```python
from build123d import *

# Parameters (mm, degrees)
SKETCH2_R           = 3
BOSS_EXTRUDE1_DEPTH = 5
SKETCH3_R           = 1.5
BOSS_EXTRUDE2_DEPTH = 5
CUT_EXTRUDE1_START  = -2.5
CUT_EXTRUDE1_DEPTH  = 2.5


with BuildPart() as part:
    # Sketch2 → Boss-Extrude1 (new body)
    with BuildSketch(Plane(origin=(0, 0, 0), x_dir=(1, 0, 0), z_dir=(0, 1, 0))):
        with Locations(Location((0, 0, 0), (0, 0, 270))):
            Circle(SKETCH2_R)
    extrude(amount=BOSS_EXTRUDE1_DEPTH)

    # Sketch3 → Boss-Extrude2 (add)
    with BuildSketch(Plane(origin=(0, 5, 0), x_dir=(1, 0, 0), z_dir=(0, 1, 0))):
        with Locations(Location((0, 0, 0), (0, 0, 270))):
            Circle(SKETCH3_R)
    extrude(amount=BOSS_EXTRUDE2_DEPTH)

    # Sketch4 → Cut-Extrude1 (cut)
    with BuildSketch(Plane(origin=(0, 10, 0), x_dir=(1, 0, 0), z_dir=(0, 1, 0)).offset(CUT_EXTRUDE1_START)):
        with BuildLine():
            Line((-1.456893676, -0.357016549), (1.456893676, -0.357016549))
            ThreePointArc((1.456893676, -0.357016549), (0, -1.5), (-1.456893676, -0.357016549))
        make_face()
    extrude(amount=CUT_EXTRUDE1_DEPTH, mode=Mode.SUBTRACT)


solid = part.part
```
Input: part model. Units: mm. Frame: model coordinates. A direction names the side the tool comes from. Round coordinates to 2 decimals unless told otherwise and drop trailing zeros. Loops run counter-clockwise (first coordinate to the right, second up) from the corner with the lowest first, then second, coordinate; pieces in that order, holes last. Notation, with made-up numbers: (11.5, 57) - (51.5, 57) arc R13 cw to (51.5, 75) - close; hole circle Ø2 at (-26, -6.75). An arc over 180 degrees is marked (long way). One line per item, written item: value. Start each with the question number.
(1) Section B-B, the plane z = 0.15. Return loops of the section in (x, y).
(2) Ray query, line 1 (Y direction, x = -2.3, z = 1.8); line 2 (Y direction, x = -0.15, z = 0.75); line 3 (Z direction, x = 2.6, y = 1). Return the intervals inside material, ascending. Write a range as [from, to].
(3) Section D-D, the plane z = -0.8. Return loops of the section in (x, y), plus the area to 3 significant figures.
(4) Access query for faces 1 (the cylindrical face through (0.07, 6.91, -1.5)), 2 (the flat face through (0, 9, 0.357)), 3 (the flat face through (0, 10, 0)). Directions: +Z, -Z, +X, -X, +Y, -Y. A direction counts if a zero-diameter tool reaches every point of the face in a straight line with its end or side. Return the directions, or none.
(5) Section C-C, the plane y = 8.5. Return loops of the section in (x, z), plus the area to 3 significant figures.
(6) Contact query for flat-ended pins moving along their axis: P1, Ø0.6, axis at x = 0, z = 1, coming from the +Y side; P2, Ø2, axis at x = 0, y = 8, coming from the +Z side. Output: stop coordinate, or through.
(7) Section A-A, the plane x = 0. Return loops of the section in (y, z).
Results below:
1. outline: (-3, 0) - (3, 0) - (3, 5) - (1.49, 5) - (1.49, 10) - (-1.49, 10) - (-1.49, 5) - (-3, 5) - close
2. line 1: [0, 5]
2. line 2: [0, 7.5]
2. line 3: [-1.5, 1.5]
3. outline: (-2.89, 0) - (2.89, 0) - (2.89, 5) - (1.27, 5) - (1.27, 10) - (-1.27, 10) - (-1.27, 5) - (-2.89, 5) - close
3. area: 41.6 mm^2
4. face 1: +Y
4. face 2: +Z, +X, -X, +Y
4. face 3: +Z, -Z, +X, -X, +Y
5. outline: (-1.46, 0.36) arc R1.5 ccw (long way) to (1.46, 0.36) - close
5. area: 4.60 mm^2
6. P1: y = 7.5
6. P2: z = 1.5
7. outline: (0, -3) - (5, -3) - (5, -1.5) - (10, -1.5) - (10, 0.36) - (7.5, 0.36) - (7.5, 1.5) - (5, 1.5) - (5, 3) - (0, 3) - close
